from build123d import *

# Parameters (mm, degrees)
BOSS_EXTRUDE1_DEPTH      = 125
BOSS_EXTRUDE1_DEPTH_BACK = 125


with BuildPart() as part:
    # Sketch1 → Boss-Extrude1 (new body, two sides)
    with BuildSketch(Plane(origin=(0, 0, 0), x_dir=(0, 1, 0), z_dir=(0, 0, 1))) as boss_extrude1_sk:
        Polygon((-14, 20), (-20, 20), (-20, 14), (-19, 13), (-18.5, 13), (-18.5, 16.292893219), (-17, 16.292893219), (-13.5, 12.792893219), (-13.5, 7.95), (-17, 4.45), (-18.5, 4.45), (-18.5, 7), (-19, 7), (-20, 6), (-20, -6), (-19, -7), (-18.5, -7), (-18.5, -4.45), (-17, -4.45), (-13.5, -7.95), (-13.5, -12.792893219), (-17, -16.292893219), (-18.5, -16.292893219), (-18.5, -13), (-19, -13), (-20, -14), (-20, -20), (-14, -20), (-13, -19), (-13, -18.5), (-16.292893219, -18.5), (-16.292893219, -17), (-12.792893219, -13.5), (-7.95, -13.5), (-4.45, -17), (-4.45, -18.5), (-7, -18.5), (-7, -19), (-6, -20), (6, -20), (7, -19), (7, -18.5), (4.45, -18.5), (4.45, -17), (7.95, -13.5), (12.792893219, -13.5), (16.292893219, -17), (16.292893219, -18.5), (13, -18.5), (13, -19), (14, -20), (20, -20), (20, -14), (19, -13), (18.5, -13), (18.5, -16.292893219), (17, -16.292893219), (13.5, -12.792893219), (13.5, -7.95), (17, -4.45), (18.5, -4.45), (18.5, -7), (19, -7), (20, -6), (20, 6), (19, 7), (18.5, 7), (18.5, 4.45), (17, 4.45), (13.5, 7.95), (13.5, 12.792893219), (17, 16.292893219), (18.5, 16.292893219), (18.5, 13), (19, 13), (20, 14), (20, 20), (14, 20), (13, 19), (13, 18.5), (16.292893219, 18.5), (16.292893219, 17), (12.792893219, 13.5), (7.95, 13.5), (4.45, 17), (4.45, 18.5), (7, 18.5), (7, 19), (6, 20), (-6, 20), (-7, 19), (-7, 18.5), (-4.45, 18.5), (-4.45, 17), (-7.95, 13.5), (-12.792893219, 13.5), (-16.292893219, 17), (-16.292893219, 18.5), (-13, 18.5), (-13, 19), align=None)
        Polygon((3.25, 16.502943725), (3.25, 18.5), (-3.25, 18.5), (-3.25, 16.502943725), (-6.5, 13.252943725), (-6.5, 6.5), (-13.252943725, 6.5), (-16.502943725, 3.25), (-18.5, 3.25), (-18.5, -3.25), (-16.502943725, -3.25), (-13.252943725, -6.5), (-6.5, -6.5), (-6.5, -13.252943725), (-3.25, -16.502943725), (-3.25, -18.5), (3.25, -18.5), (3.25, -16.502943725), (6.5, -13.252943725), (6.5, -6.5), (13.252943725, -6.5), (16.502943725, -3.25), (18.5, -3.25), (18.5, 3.25), (16.502943725, 3.25), (13.252943725, 6.5), (6.5, 6.5), (6.5, 13.252943725), align=None, mode=Mode.SUBTRACT)
        with BuildLine():
            ThreePointArc((-8.585786438, 8.585786438), (-8.585786438, 11.414213562), (-11.414213562, 11.414213562))
            ThreePointArc((-11.414213562, 11.414213562), (-11.414213562, 8.585786438), (-8.585786438, 8.585786438))
        make_face(mode=Mode.SUBTRACT)
        with BuildLine():
            ThreePointArc((8.585786438, 8.585786438), (8.585786438, 11.414213562), (11.414213562, 11.414213562))
            ThreePointArc((11.414213562, 11.414213562), (11.414213562, 8.585786438), (8.585786438, 8.585786438))
        make_face(mode=Mode.SUBTRACT)
        with BuildLine():
            ThreePointArc((8.585786438, -8.585786438), (11.414213562, -8.585786438), (11.414213562, -11.414213562))
            ThreePointArc((11.414213562, -11.414213562), (8.585786438, -11.414213562), (8.585786438, -8.585786438))
        make_face(mode=Mode.SUBTRACT)
        with BuildLine():
            ThreePointArc((-8.585786438, -8.585786438), (-8.585786438, -11.414213562), (-11.414213562, -11.414213562))
            ThreePointArc((-11.414213562, -11.414213562), (-11.414213562, -8.585786438), (-8.585786438, -8.585786438))
        make_face(mode=Mode.SUBTRACT)
    extrude(amount=BOSS_EXTRUDE1_DEPTH)
    extrude(boss_extrude1_sk.sketch, amount=-BOSS_EXTRUDE1_DEPTH_BACK)


solid = part.part
Source: CAD feature listing. Evaluate the final solid. Frame: model axes, mm. A direction names the side the tool comes from. Coordinates: 2 decimals unless noted, no trailing zeros. Answer in a Markdown table with one row per item. Add a question column.
Q1. Section A-A on z = 32. Give the number of separate pieces and of enclosed holes in the cut face, and give its area (3 significant figures).
Q2. Pull-direction query (X, two-part tool) for faces 4 (the face through (-20, 0, 2)), 5 (the face through (-10, -13.5, 2)), 6 (the face through (13.5, -10, 2)); classes: pulls with the +X half, pulls with the -X half, needs draft (parallel to the pull), parting line crosses it, or undercut.
Q3. Reachability of faces 1 (the face through (13.5, 10, 2)), 2 (the face through (-13.5, 10, 2)), 3 (the face through (10, 13.5, 2)) from +Z, -Z, +X, -X, +Y, -Y: full face, straight path, thin tool, end or side. Return the list, or none.
Q4. Ray query, line 1 along Y through (x, z) = (-10, 93); line 2 along Y through (x, z) = (17, 86). Return the intervals inside material, ascending.
Q5. Contact query for flat-ended pins moving along their axis: pin 1 Ø5.5 at (y, z) = (-11, 67.5) entering from +X; pin 2 Ø5 at (x, y) = (5.5, 5.5) entering from -Z. Output: stop coordinate, or through.
Computed values:
| question | item | result |
|---|---|---|
| 1 | separate pieces | 1 |
| 1 | enclosed holes | 5 |
| 1 | area | 395 mm^2 |
| 2 | face 4 | pulls with the -X half |
| 2 | face 5 | undercut |
| 2 | face 6 | pulls with the +X half |
| 3 | face 1 | +Z, -Z, +X |
| 3 | face 2 | +Z, -Z, -X |
| 3 | face 3 | +Z, -Z, +Y |
| 4 | line 1 | y = -13.5 to -12, -8 to -6.5, 6.5 to 8, 12 to 13.5 |
| 4 | line 2 | y = -20 to -16.29, -4.45 to -3.25, 3.25 to 4.45, 16.29 to 20 |
| 5 | pin 1 | stops at x = 19.75 |
| 5 | pin 2 | stops at z = -125 |
